Check sheet for the modelled part. Datum: model origin and axes. Units: mm. A direction names the side the tool comes from. Round coordinates to 2 decimals unless told otherwise and drop trailing zeros. Write each loop counter-clockwise with the first axis right and the second up, starting at its lowest first coordinate (ties: lowest second). Pieces come first, ordered by that corner, then holes.
Autodesk Inventor part; units mm, degrees
ref_plane "YZ Plane" through (0, 0, 0) normal (1, 0, 0) x (0, 1, 0)
ref_plane "XZ Plane" through (0, 0, 0) normal (0, 1, 0) x (-1, 0, 0)
ref_plane "XY Plane" through (0, 0, 0) normal (0, 0, 1) x (1, 0, 0)
sketch "草圖1" plane through (0, 0, 0) normal (0, 0, 1) x (1, 0, 0)
  line L0 (0, 0) -> (-34.5, 0)
  line L1 (-34.5, 0) -> (-34.5, -0.8)
  line L2 (-34.5, -0.8) -> (0, -0.8)
  line L3 (0, -0.8) -> (0, 0)
  line L4 (0, -0.8) -> (-31.5, -0.8)
  line L5 (-31.5, -0.8) -> (-31.5, -10)
  line L6 (-31.5, -10) -> (0, -10)
  line L7 (0, -10) -> (0, -0.8)
  line L8 (0, -10) -> (-30, -10)
  line L9 (-30, -10) -> (-30, -12)
  line L10 (-30, -12) -> (0, -12)
  line L11 (0, -12) -> (0, -10)
  line L12 (-18.0931, -47) -> (0, -47)
  line L13 (0, -47) -> (0, -12)
  line L14 (0, -47) -> (-20, -47)
  line L15 (-20, -47) -> (-20, -50)
  line L16 (-20, -50) -> (0, -50)
  line L17 (0, -50) -> (0, -47)
  line L18 (0, -50) -> (-19.9, -50)
  line L19 (-19.9, -50) -> (-19.9, -55)
  line L20 (-19.9, -55) -> (0, -55)
  line L21 (0, -55) -> (0, -50)
  line L22 (0, -47) -> (-27, -47)
  line L23 (-27, -47) -> (-28.5, -12)
  dimension "d0" = 0.8
  dimension "d1" = 34.5
  dimension "d2" = 20
  dimension "d3" = 31.5
  dimension "d4" = 30
  dimension "d5" = 9.2
  dimension "d6" = 2
  dimension "d8" = 3
  dimension "d9" = 28.5
  dimension "d10" = 27
  dimension "d11" = 19.9
  dimension "d12" = 35
  dimension "d13" = 5
revolve "迴轉1" add sketch "草圖1" angle 360 about axis through (0, -47, 0) along (0, 1, 0) contours L3 L2 L1 L0 | L7 L6 L5 L2 | L11 L10 L9 L6 | L13 L12 L14 L22 L23 L10
fillet "圓角1" radius 10 1 edges at (27, -47, 0)
shell "薄殼1" thickness 1 removed faces 1 at (11.3362, 0, -5.1612)
properties part number "布丁"
1. Sectioned sample at A-A, the plane y = -33. Enter the section's corners in (x, z).
2. Go/stop test with flat-tipped pins: pin 1 (10 mm diameter, centred on y = -24.5, z = 21.5, fed in from -X); pin 2 (6 mm diameter, centred on y = -36.5, z = -11, fed in from +X); pin 3 (1.5 mm diameter, centred on y = -8, z = -19, fed in from -X). Record where each tip stops, or that it passes through.
3. Scan lines: line 1 along Z through (x, y) = (0, -6.5); line 2 along Z through (x, y) = (0, -10.45); line 3 along X through (y, z) = (-6.5, 1.5). Record each from-to range of solid material in increasing order.
4. Set-up check for faces 1 (the flat face through (0, 0, -31)), 2 (the flat face through (-15, -0.8, -28)), 3 (the cylindrical face through (-28.174, -4.563, 11.681)): record each of +Z, -Z, +X, -X, +Y, -Y from which the full face is reachable in a straight line by a thin tool's end or side.
5. Release check for a two-part mould opening along Z. For faces 4 (the flat face through (-11, -12, -27)), 5 (the cylindrical face through (4.101, -5.464, -31.232)), 6 (the flat face through (-11, -9, -27)) record: released by +Z, released by -Z, zero draft, split by the parting line, or undercut.
Computed values:
1. outline: circle Ø55.2 at (0, 0); hole circle Ø53.2 at (0, 0)
2. pin 1: stops at x = -22.59
2. pin 2: stops at x = 26.27
2. pin 3: stops at x = -25.67
3. line 1: z = -31.5 to -30.5, 30.5 to 31.5
3. line 2: z = -30 to -29, 29 to 30
3. line 3: x = -31.46 to -30.46, 30.46 to 31.46
4. face 1: +Z, -Z, +X, -X, +Y
4. face 2: -Y
4. face 3: +Y
5. face 4: zero draft
5. face 5: split by the parting line
5. face 6: undercut
